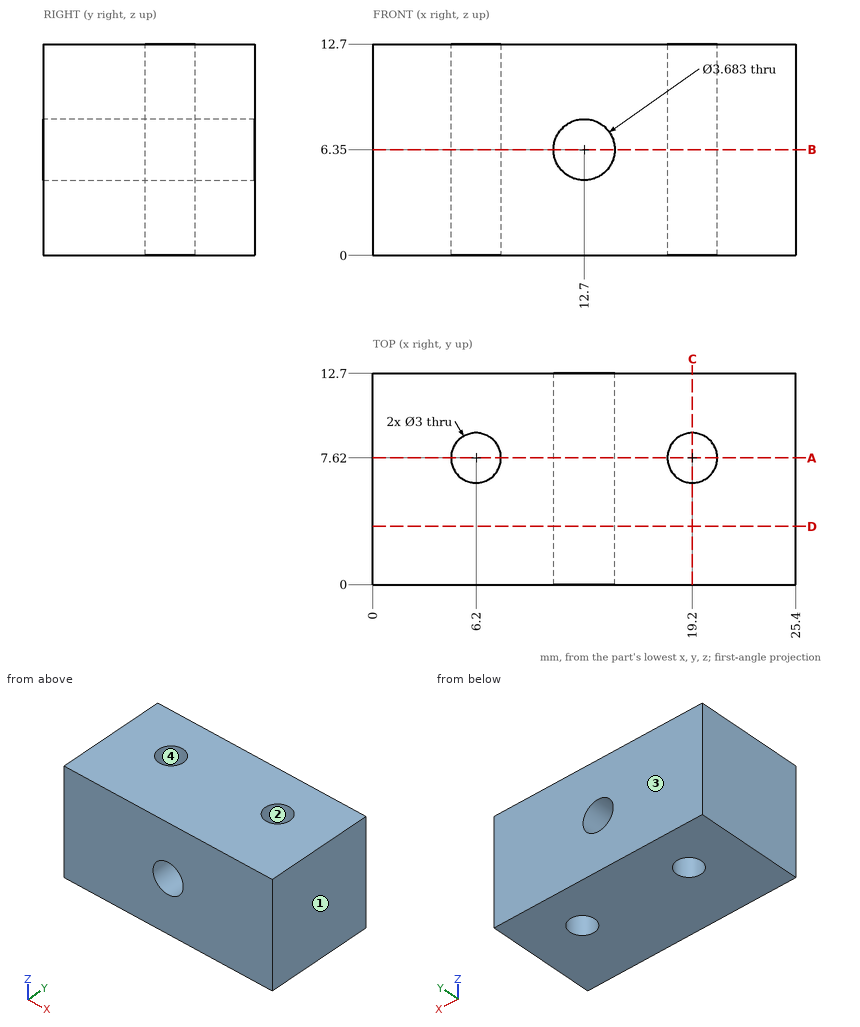
Job drawing, mm, ordinate dimensions from the low corner. One solid piece. Give positions to 0.01 mm unless a question says otherwise; leave off trailing zeros. Loops run counter-clockwise (first coordinate to the right, second up) from the corner with the lowest first, then second, coordinate; pieces in that order, holes last. Notation, with made-up numbers: (67, -13.5) -> (115, -13.5) arc R19 cw to (115, -9.5) -> close; hole circle Ø8 at (75.25, 58.5). An arc over 180 degrees is marked (long way). Use a Markdown table: item, result. Add a question column.
(1) Slice it at C-C on x = 19.2. List the corners of the cut face in (y, z).
(2) Slice it at B-B on z = 6.35. List the corners of the cut face in (x, y).
(3) Slice it at A-A on y = 7.62. List the corners of the cut face in (x, z).
(4) Slice it at D-D on y = 3.5. List the corners of the cut face in (x, z), and give its area (3 significant figures).
(5) Wall check: line 1 along X through (y, z) = (7.75, 10.25); line 2 along Y through (x, z) = (19.2, 5.5); line 3 along X through (y, z) = (9.5, 6.35). Give the ranges that are in metal, low to high.
(6) Mould opens along Y. For the marked faces 1, 2, 3 and 4 say: +Y half, -Y half, draft (parallel to the pull), parting line (faces both ways), or undercut.
Filled sheet:
| question | item | result |
|---|---|---|
| 1 | outline | (0, 0) -> (6.12, 0) -> (6.12, 12.7) -> (0, 12.7) -> close; (9.12, 0) -> (12.7, 0) -> (12.7, 12.7) -> (9.12, 12.7) -> close |
| 2 | outline | (0, 0) -> (10.86, 0) -> (10.86, 12.7) -> (0, 12.7) -> close; (14.54, 0) -> (25.4, 0) -> (25.4, 12.7) -> (14.54, 12.7) -> close; hole circle Ø3 at (6.2, 7.62); hole circle Ø3 at (19.2, 7.62) |
| 3 | outline | (0, 0) -> (4.7, 0) -> (4.7, 12.7) -> (0, 12.7) -> close; (7.7, 0) -> (17.7, 0) -> (17.7, 12.7) -> (7.7, 12.7) -> close; (20.7, 0) -> (25.4, 0) -> (25.4, 12.7) -> (20.7, 12.7) -> close; hole circle Ø3.68 at (12.7, 6.35) |
| 4 | outline | (0, 0) -> (25.4, 0) -> (25.4, 12.7) -> (0, 12.7) -> close; hole circle Ø3.68 at (12.7, 6.35) |
| 4 | area | 312 mm2 |
| 5 | line 1 | 0 to 4.71, 7.69 to 17.71, 20.69 to 25.4 |
| 5 | line 2 | 0 to 6.12, 9.12 to 12.7 |
| 5 | line 3 | 0 to 10.86, 14.54 to 25.4 |
| 6 | face 1 | draft |
| 6 | face 2 | undercut |
| 6 | face 3 | +Y half |
| 6 | face 4 | undercut |
